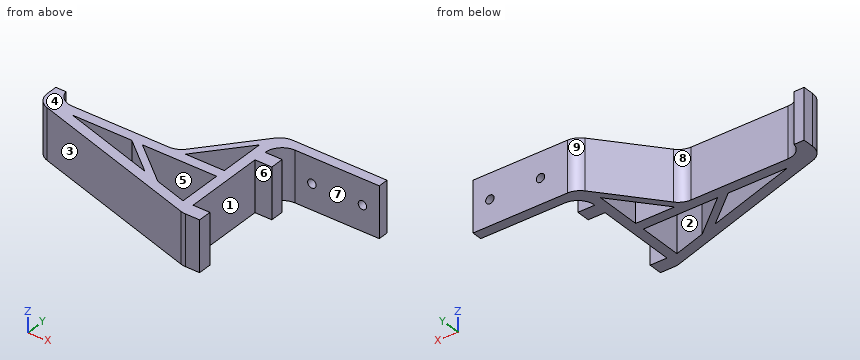
from build123d import *

# Parameters (mm, degrees)
F1_DEPTH    = 15
F2_R        = 1.25
F3_DEPTH    = 40.1383324758
F4_R        = 5
F5_W        = 4
F5_H        = 15
F6_DEPTH    = 5
F8_DEPTH    = 15
F9_T1_DEPTH = 15
F9_T3_DEPTH = 15
F9_T5_DEPTH = 33.4938424429
F9_T7_DEPTH = 18.7397003757


# Not quite as in the source:
# - a fillet or chamfer that OpenCascade refuses, or shapes differently, is made with other operations: its cross-section is extruded or revolved along the edge and cut away or added


with BuildPart() as f1:
    # F0 (on Top) → F1 (new body)
    with BuildSketch(Plane.XY):
        Polygon((0, 20), (0, 23), (-33, 23), (-33, 3), (-83, 3), (-83, 7), (-86, 7), (-86, 0), (-30, -17.1373324758), (-30, -14), (-30, 0), (-30, 20), align=None)
        Polygon((-47.7579661467, -8.5656398223), (-75.7480766687, 0), (-58.1432454597, 0), align=None, mode=Mode.SUBTRACT)
        Polygon((-33, 0), (-33, -13.0819286174), (-42.760486377, -10.0949875429), (-55, 0), align=None, mode=Mode.SUBTRACT)
    extrude(amount=F1_DEPTH)

    # F2 (on face) → F3 (cut, through all)
    with BuildSketch(Plane(origin=(0, 23, 0), x_dir=(-1, 0, 0), z_dir=(0, 1, 0))):
        with Locations((5, 7.5)):
            Circle(F2_R)
        with Locations((20, 7.5)):
            Circle(F2_R)
    extrude(amount=-F3_DEPTH, mode=Mode.SUBTRACT)

    # F4
    f4_edges = [f1.edges().sort_by_distance(p)[0] for p in [
        (-33, 23, 7.5),
        (-30, 20, 7.5),
    ]]
    fillet(f4_edges, radius=F4_R)

    # F5 (on face) → F6 (join)
    with BuildSketch(Plane.YZ.offset(-30)):
        with Locations((-15.1373324758, 7.5)):
            Rectangle(F5_W, F5_H)
        with Locations((13, 7.5)):
            Rectangle(F5_W, F5_H)
    extrude(amount=F6_DEPTH)

    # F7 (on face) → F8 (join, through all)
    with BuildSketch(Plane.XY.offset(15)):
        with BuildLine():
            Line((-31.8302222156, 21.2139380484), (-47.1135309143, 3))
            Line((-47.1135309143, 3), (-44.5027163357, 3))
            Line((-44.5027163357, 3), (-33, 16.7084035176))
            Line((-33, 16.7084035176), (-33, 18))
            ThreePointArc((-33, 18), (-32.6984631039, 19.7101007166), (-31.8302222156, 21.2139380484))
        make_face()
    extrude(amount=-F8_DEPTH)

    # F9: fillet of radius 5 on 4 edges, made by hand

    # F9_s2 → F9_t1 (join)
    with BuildSketch(Plane.XY):
        with BuildLine():
            ThreePointArc((-78.1010205144, 3), (-81.2632981746, 4.1270166538), (-83, 7))
            Line((-83, 7), (-83, 3))
            Line((-83, 3), (-78.1010205144, 3))
        make_face()
    extrude(amount=F9_T1_DEPTH)

    # F9_s4 → F9_t3 (join)
    with BuildSketch(Plane.XY):
        with BuildLine():
            ThreePointArc((-45.6148469895, 4.7860619516), (-47.3319778964, 3.4684610648), (-49.4450692051, 3))
            Line((-49.4450692051, 3), (-47.1135309143, 3))
            Line((-47.1135309143, 3), (-45.6148469895, 4.7860619516))
        make_face()
    extrude(amount=F9_T3_DEPTH)

    # F9_s6 → F9_t5 (cut)
    with BuildSketch(Plane.XY.offset(-9.2469212215)):
        with BuildLine():
            ThreePointArc((-86, 3.6987684886), (-85.0196828505, 0.7251932363), (-82.4631400875, -1.08236329))
            Line((-82.4631400875, -1.08236329), (-86, 0))
            Line((-86, 0), (-86, 3.6987684886))
        make_face()
    extrude(amount=F9_T5_DEPTH, mode=Mode.SUBTRACT)

    # F9_s8 → F9_t7 (cut)
    with BuildSketch(Plane.XY.offset(-1.8698501879)):
        with BuildLine():
            ThreePointArc((-29.2520599249, -17.1373324758), (-29.9917697014, -17.0823127029), (-30.7152000124, -16.9184642544))
            Line((-30.7152000124, -16.9184642544), (-30, -17.1373324758))
            Line((-30, -17.1373324758), (-29.2520599249, -17.1373324758))
        make_face()
    extrude(amount=F9_T7_DEPTH, mode=Mode.SUBTRACT)


solid = f1.part
Source: CAD feature listing. Evaluate the final solid. Frame: model axes, mm. Face numbers are marked on the shaded views. A direction names the side the tool comes from. Round coordinates to 2 decimals unless told otherwise and drop trailing zeros. Write each loop counter-clockwise with the first axis right and the second up, starting at its lowest first coordinate (ties: lowest second). Pieces come first, ordered by that corner, then holes. Notation, with made-up numbers: M 78,76 L 110,76 A9 ccw 110,84 Z; hole C 10.25,78.25 d5. An arc over 180 degrees is marked long. One line per item, written item: value. Start each with the question number.
Item 1: Section query C-C (y = -12). Return the cut outline in (x, z).
Item 2: Mould query, pull axis X, two halves, no side actions, for the marked faces 1, 2, 3 and 4. Classes: pulls with the +X half, pulls with the -X half, needs draft (parallel to the pull), parting line crosses it, or undercut.
Item 3: Section query A-A (x = -5). Return the cut outline in (y, z), plus the area to 3 significant figures.
Item 4: Section query D-D (x = -37). Return the cut outline in (y, z), plus the area to 3 significant figures.
Item 5: Pin query (flat end, axial travel): pin 1 (3 mm diameter, centred on y = 14, z = 11.5, fed in from -X); pin 2 (2 mm diameter, centred on y = 16, z = 4, fed in from -X); pin 3 (4.5 mm diameter, centred on x = -66.5, z = 5, fed in from -Y). Return the tip coordinate at first contact, or that it passes through.
Item 6: Set-up query: the marked faces 5, 6, 7, 8 and 9. Return all of +Z, -Z, +X, -X, +Y, -Y with unobstructed straight access to the full face (end or side cutting, diameter ignored); none if empty.
Item 7: Ray query, L1, parallel to Z at x = -20, y = 21.5; L2, parallel to Y at x = -49, z = 12; L3, parallel to Y at x = -7.5, z = 8. Return the intervals inside material, ascending. Write a range as from..to.
Item 8: Section query B-B (z = 10.25). State how many separate pieces and enclosed holes the cut face has, plus the area to 3 significant figures.
Result set:
1. outline: M -46.79,0 L -36.54,0 L -36.54,15 L -46.79,15 Z; M -33,0 L -30,0 L -30,15 L -33,15 Z
2. face 1: pulls with the +X half
2. face 2: undercut
2. face 3: pulls with the -X half
2. face 4: needs draft
3. outline: M 20,0 L 23,0 L 23,6.25 L 20,6.25 Z; M 20,8.75 L 23,8.75 L 23,15 L 20,15 Z
3. area: 37.5 mm²
4. outline: M -15,0 L -11.86,0 L -11.86,15 L -15,15 Z; M 0,0 L 3,0 L 3,15 L 0,15 Z; M 11.94,0 L 15.05,0 L 15.05,15 L 11.94,15 Z
4. area: 139 mm²
5. pin 1: stops at x = -39.14
5. pin 2: stops at x = -37.04
5. pin 3: stops at y = -6.66
6. face 5: +Z, -Z
6. face 6: +Z, -Z, +X
6. face 7: +Z, -Z, +X, -Y
6. face 8: +Z, -Z, +Y
6. face 9: +Z, -Z, -X, +Y
7. L1: z = 0..6.25, 8.75..15
7. L2: y = -11.32..-8.19, -7.54..-4.95, 0..3.02
7. L3: y = 20..23
8. separate pieces: 1
8. enclosed holes: 3
8. area: 643 mm²
